Geometry check sheet. Reference: the model listing, model coordinates, mm. A direction names the side the tool comes from. Coordinates: 2 decimals unless noted, no trailing zeros. Loops run counter-clockwise (first coordinate to the right, second up) from the corner with the lowest first, then second, coordinate; pieces in that order, holes last.
Autodesk Inventor part; units mm, degrees
ref_plane "YZ Plane" through (0, 0, 0) normal (1, 0, 0) x (0, 1, 0)
ref_plane "XZ Plane" through (0, 0, 0) normal (0, 1, 0) x (-1, 0, 0)
ref_plane "XY Plane" through (0, 0, 0) normal (0, 0, 1) x (1, 0, 0)
sketch "Sketch1" plane through (0, 0, 0) normal (0, 0, 1) x (1, 0, 0)
  line L0 (-24.5, 26) -> (24.5, 26)
  line L1 (24.5, 26) -> (24.5, -26)
  line L2 (24.5, -26) -> (-24.5, -26)
  line L3 (-24.5, -26) -> (-24.5, 26)
  point P0 (0, 0)
  dimension "d0" = 52
  dimension "d1" = 26
  dimension "d2" = 49
  dimension "d3" = 24.5
extrude "Extrusion1" add sketch "Sketch1" along normal blind 11.55
sketch "Sketch3" plane through (0, 0, 11.55) normal (0, 0, 1) x (1, 0, 0)
  line L0 (-24.5, -26) -> (24.5, -26)
  line L1 (0, -26) -> (0, -20.5)
  line L2 (24.5, 26) -> (-24.5, 26)
  line L3 (0, 26) -> (0, 20.5)
  point P0 (0, 0)
  point P1 (0, 0)
  dimension "d13" = 5.5
  dimension "d14" = 20.5
  dimension "d15" = 5.5
  dimension "d16" = 20.5
hole "Hole1" at (0, 20.5, 11.55) at (0, -20.5, 11.55) direction (0, 0, -1) diameter 4.305 depth 12.3 counterbore diameter 7.938 counterbore depth 2.4
sketch "Sketch5" plane through (0, 0, 0) normal (0, 0, -1) x (-1, 0, 0)
  line L0 (-24.5, 26) -> (24.5, 26)
  line L1 (24.5, 26) -> (24.5, -26)
  point P0 (0, 0)
  point P1 (0, 0)
  dimension "d31" = 26
  dimension "d32" = 24.5
hole "Hole3" at (0, 0, 0) direction (0, 0, 1) diameter 4.5 depth 11.8 counterbore diameter 8 counterbore depth 4
fillet "Fillet1" radius 2 4 edges at (-24.5, -26, 5.775) (-24.5, 26, 5.775) (24.5, -26, 5.775) (24.5, 26, 5.775)
sketch "Sketch7" plane through (-24.5, -24, 0) normal (-1, 0, 0) x (0, 0, 1)
  circle A0 centre (-12.35, 24) radius 12.7
  point P0 (0, 24)
  dimension "d57" = 25.4
  dimension "d58" = 12.35
extrude "Extrusion3" cut sketch "Sketch7" against normal blind 50
sketch "Sketch10" plane through (0, 0, 0) normal (0, 0, -1) x (-1, 0, 0)
  circle A0 centre (0, 0) radius 1.621
  line L0 (0, 0) -> (-18.5, 0)
  line L1 (-18.5, 0) -> (-18.5, -7.5)
  line L2 (-18.5, -7.5) -> (0, -7.5)
  line L3 (0, -7.5) -> (0, 0)
  point P0 (-18.5, 7.5)
  point P1 (18.5, 7.5)
  point P2 (18.5, -7.5)
  dimension "d77" = 18.5
  dimension "d78" = 7.5
  dimension "d79" = 18.5
  dimension "d80" = 37
  dimension "d81" = 18.5
  dimension "d82" = 7.5
  dimension "d83" = 7.5
  dimension "d84" = 7.5
hole "Hole5" at (18.5, -7.5, 0) at (18.5, 7.5, 0) at (-18.5, 7.5, 0) at (-18.5, -7.5, 0) direction (0, 0, 1) diameter 2.9 end through all counterbore diameter 5.5 counterbore depth 7.5
equation "\"d15\" = d13"
properties part number "ADAPTER_EOM14.7GHz_new"
(1) Scan lines: L1, parallel to Y at x = 18.5, z = 5.25; L2, parallel to Y at x = 0, z = 10.7; L3, parallel to X at y = 7.5, z = 9.7. Record each from-to range of solid material in increasing order.
Findings:
L1: y = -26 to -10.25, -4.75 to 4.75, 10.25 to 26
L2: y = -26 to -24.47, -16.53 to -2.25, 2.25 to 16.53, 24.47 to 26
L3: x = -24.5 to -19.95, -17.05 to 17.05, 19.95 to 24.5
(2) Sectioned sample at A-A on y = 0. Record the cut outline in (x, z).
Findings:
outline: (-24.5, 0.35) - (-4, 0.35) - (-4, 4) - (-2.25, 4) - (-2.25, 11.55) - (-24.5, 11.55) - close; (2.25, 4) - (4, 4) - (4, 0.35) - (24.5, 0.35) - (24.5, 11.55) - (2.25, 11.55) - close
(3) Sectioned sample at B-B on x = 0. Record the cut outline in (y, z).
Findings:
outline: (-26, 0) - (-22.65, 0) - (-22.65, 9.15) - (-24.47, 9.15) - (-24.47, 11.55) - (-26, 11.55) - close; (-18.35, 0) - (-4, 0) - (-4, 4) - (-2.25, 4) - (-2.25, 11.55) - (-16.53, 11.55) - (-16.53, 9.15) - (-18.35, 9.15) - close; (2.25, 4) - (4, 4) - (4, 0) - (18.35, 0) - (18.35, 9.15) - (16.53, 9.15) - (16.53, 11.55) - (2.25, 11.55) - close; (22.65, 0) - (26, 0) - (26, 11.55) - (24.47, 11.55) - (24.47, 9.15) - (22.65, 9.15) - close
(4) Sectioned sample at D-D on x = 18.5. Record the cut outline in (y, z), and give its area (3 significant figures).
Findings:
outline: (-26, 0) - (-10.25, 0) - (-10.25, 7.5) - (-8.95, 7.5) - (-8.95, 11.55) - (-26, 11.55) - close; (-6.05, 7.5) - (-4.75, 7.5) - (-4.75, 0) - (-2.96, 0) arc R12.7 cw to (2.96, 0) - (4.75, 0) - (4.75, 7.5) - (6.05, 7.5) - (6.05, 11.55) - (-6.05, 11.55) - close; (8.95, 7.5) - (10.25, 7.5) - (10.25, 0) - (26, 0) - (26, 11.55) - (8.95, 11.55) - close
area: 493 mm2
(5) Draft check along Y on faces 1 (the cylindrical face through (-23.93, -25.4, 5.86)), 2 (the flat face through (24.5, 0, 6)), 3 (the cylindrical face through (19.38, 6.35, 9.55)). Enter one of: +Y half, -Y half, draft (parallel to the pull), parting line (faces both ways), or undercut.
Findings:
face 1: -Y half
face 2: draft
face 3: undercut
(6) Access from +Z, -Z, +X, -X, +Y, -Y to the whole of each face (thin tool, end or side, straight path). Record for faces 4 (the cylindrical face through (-17.62, 6.35, 9.55)), 5 (the cylindrical face through (-1.192, -24.286, 10.333)), 6 (the flat face through (20, -6, 7.5)).
Findings:
face 4: +Z, -Z
face 5: +Z
face 6: -Z
(7) Gauge pin test, flat ends, axial feed: pin 1 Ø6.5 at (x, y) = (0, 0) entering from -Z; pin 2 Ø3 at (x, y) = (-18, 6.5) entering from -Z. Record the tip position at first contact, or that the pin passes through.
Findings:
pin 1: stops at z = 4
pin 2: stops at z = 7.5
(8) Sectioned sample at C-C on z = 5.75. State how many separate pieces and enclosed holes the cut face has, and give its area (3 significant figures).
Findings:
separate pieces: 1
enclosed holes: 7
area: 2,400 mm2
